Part model, mm, in its own coordinate system. A direction names the side the tool comes from. Coordinates: 2 decimals unless noted, no trailing zeros. Order: outer loops, then holes, each group sorted by start corner. A loop starts at its lowest first (then second) coordinate and runs counter-clockwise, first axis right, second up. Notation, with made-up numbers: (3.5, 42) - (51.5, 42) arc R22 cw to (51.5, 80) - close; hole circle Ø1 at (60.5, 70.25). An arc over 180 degrees is marked (long way). Use a Markdown table: item, result. Add a question column.
1) Saw through at A-A on y = 0. List the corners of the cut face in (x, z), then the cut area to 3 significant figures.
2) Saw through at C-C on x = 12.5. List the corners of the cut face in (y, z).
3) Saw through at B-B on z = 10.5. List the corners of the cut face in (x, y), then the cut area to 3 significant figures.
4) Wall check: L1, parallel to Z at x = -25.2, y = 0; L2, parallel to Y at x = -12, z = 5.25; L3, parallel to Y at x = 7, z = 8.75. Give the ranges that are in metal, low to high. Write a range as [from, to].
5) Saw through at D-D on y = -4.25. List the corners of the cut face in (x, z), then the cut area to 3 significant figures.
6) Tool access for faces 1 (the face through (-24, 2, 4)), 2 (the face through (24, 2, 11)), 3 (the face through (0, -7, 7)): list every direction of +Z, -Z, +X, -X, +Y, -Y with a clear straight run to the whole face (end or side of a thin tool).
7) Two-plate mould, pull along Y, no slides. Class faces 4 (the face through (0, -1, 15)), 5 (the face through (0, 7, 7)), 6 (the face through (-25.972, -0.651, 2.543)): +Y half, -Y half, draft (parallel to the pull), parting line (faces both ways), or undercut.
8) Drop flat-ended pins along their axis: P1, Ø8, axis at y = 0, z = 7.5, coming from the +X side; P2, Ø5, axis at y = -2.5, z = 9.5, coming from the +X side. Give the stop position or say it passes through.
```python
from build123d import *

# Parameters (mm, degrees)
SKETCH1_W                = 56
SKETCH1_H                = 14
BOSS_EXTRUDE1_DEPTH      = 15
F_3_0_3_DIAMETER_HOLE1_D = 7.5
SKETCH5_R                = 5
CUT_EXTRUDE1_DEPTH       = 4
CUT_EXTRUDE2_START       = -4
SKETCH6_R                = 5
CUT_EXTRUDE2_DEPTH       = 4
FILLET1_R                = 3


with BuildPart() as part:
    # Sketch1 → Boss-Extrude1 (new body)
    with BuildSketch(Plane.XY):
        Rectangle(SKETCH1_W, SKETCH1_H)
    extrude(amount=BOSS_EXTRUDE1_DEPTH)

    # Ø3.0 (3) Diameter Hole1 (through all)
    with Locations(Plane(origin=(28, 0, 0), x_dir=(0, 0, -1), z_dir=(1, 0, 0))):
        with Locations((-7.5, 0)):
            Hole(F_3_0_3_DIAMETER_HOLE1_D / 2)

    # Sketch5 → Cut-Extrude1 (cut)
    with BuildSketch(Plane(origin=(28, 0, 0), x_dir=(0, 0, -1), z_dir=(1, 0, 0))):
        with Locations(Location((-7.5, 0, 0), (0, 0, 90))):
            Circle(SKETCH5_R)
    extrude(amount=-CUT_EXTRUDE1_DEPTH, mode=Mode.SUBTRACT)

    # Sketch6 → Cut-Extrude2 (cut)
    with BuildSketch(Plane.ZY.offset(28).offset(CUT_EXTRUDE2_START)):
        with Locations(Location((7.5, 0, 0), (0, 0, 90))):
            Circle(SKETCH6_R)
    extrude(amount=CUT_EXTRUDE2_DEPTH, mode=Mode.SUBTRACT)

    # Fillet1
    fillet1_edges = [part.edges().sort_by_distance(p)[0] for p in [
        (0, 7, 15),
        (0, 7, 0),
    ]]
    fillet(fillet1_edges, radius=FILLET1_R)


solid = part.part
```
Results are:
| question | item | result |
|---|---|---|
| 1 | outline | (-28, 0) - (28, 0) - (28, 2.5) - (24, 2.5) - (24, 3.75) - (-24, 3.75) - (-24, 2.5) - (-28, 2.5) - close; (-28, 12.5) - (-24, 12.5) - (-24, 11.25) - (24, 11.25) - (24, 12.5) - (28, 12.5) - (28, 15) - (-28, 15) - close |
| 1 | area | 400 mm2 |
| 2 | outline | (-7, 0) - (4, 0) arc R3 ccw to (7, 3) - (7, 12) arc R3 ccw to (4, 15) - (-7, 15) - close; hole circle Ø7.5 at (0, 7.5) |
| 3 | outline | (-28, -7) - (28, -7) - (28, -4) - (24, -4) - (24, -2.25) - (-24, -2.25) - (-24, -4) - (-28, -4) - close; (-28, 4) - (-24, 4) - (-24, 2.25) - (24, 2.25) - (24, 4) - (28, 4) - (28, 7) - (-28, 7) - close |
| 3 | area | 504 mm2 |
| 4 | L1 | [0, 2.5], [12.5, 15] |
| 4 | L2 | [-7, -3], [3, 7] |
| 4 | L3 | [-7, -3.54], [3.54, 7] |
| 5 | outline | (-28, 0) - (28, 0) - (28, 4.87) - (24, 4.87) - (24, 10.13) - (28, 10.13) - (28, 15) - (-28, 15) - (-28, 10.13) - (-24, 10.13) - (-24, 4.87) - (-28, 4.87) - close |
| 5 | area | 798 mm2 |
| 6 | face 1 | -X |
| 6 | face 2 | +X |
| 6 | face 3 | +Z, -Z, +X, -X, -Y |
| 7 | face 4 | draft |
| 7 | face 5 | +Y half |
| 7 | face 6 | undercut |
| 8 | P1 | x = 24 |
| 8 | P2 | x = 28 |
